Model file for the job. Use its own axes, mm. A direction names the side the tool comes from. Round coordinates to 2 decimals unless told otherwise and drop trailing zeros. Order: outer loops, then holes, each group sorted by start corner. A loop starts at its lowest first (then second) coordinate and runs counter-clockwise, first axis right, second up. Notation, with made-up numbers: (43, -24.75) - (50, -24.75) arc R24 ccw to (50, -13.75) - close; hole circle Ø8 at (45.5, 10). An arc over 180 degrees is marked (long way). Write item = value, one per line.
```python
from build123d import *

# Parameters (mm, degrees)
ESQUISSE1_W               = 47
ESQUISSE1_H               = 23
BOSS_EXTRU_1_DEPTH        = 7.071067812
TROU_TARAUD_M1_4X0_32_D   = 1.1
ESQUISSE5_W               = 20
ESQUISSE5_H               = 15
ENL_V_MAT_EXTRU_1_DEPTH   = 7.071067812
ESQUISSE6_W               = 20
ESQUISSE6_H               = 10.927419914
BOSS_EXTRU_2_DEPTH        = 7.071067812
ESQUISSE9_W               = 7.071067812
ESQUISSE9_H               = 7.071067812
BOSS_EXTRU_5_DEPTH        = 27
ESQUISSE10_R              = 1.5
ENL_V_MAT_EXTRU_2_DEPTH   = 3
TROU_TARAUD_M5X0_81_D     = 4.2
TROU_TARAUD_M5X0_81_DEPTH = 15
TROU_TARAUD_M5X0_81_TIP   = 1.2618073


with BuildPart() as part:
    # Esquisse1 → Boss.-Extru.1 (new body)
    with BuildSketch(Plane.XY):
        Rectangle(ESQUISSE1_W, ESQUISSE1_H)
    extrude(amount=BOSS_EXTRU_1_DEPTH)

    # Trou taraudé M1.4x0.32 (through all)
    with Locations(Plane(origin=(-21, 8.5, 7.071067812), x_dir=(1, 0, 0), z_dir=(0, 0, 1))):
        with Locations((0, 0), (0, -17), (42, -17), (42, 0)):
            Hole(TROU_TARAUD_M1_4X0_32_D / 2)

    # Esquisse5 → Enlèv. mat.-Extru.1 (cut)
    with BuildSketch(Plane.XY.offset(7.071067812)):
        with Locations((0, -6.927419914)):
            Rectangle(ESQUISSE5_W, ESQUISSE5_H)
    extrude(amount=-ENL_V_MAT_EXTRU_1_DEPTH, mode=Mode.SUBTRACT)

    # Esquisse6 → Boss.-Extru.2 (add)
    with BuildSketch(Plane(origin=(0, 0, 0), x_dir=(-1, 0, 0), z_dir=(0, 0, -1))):
        with Locations((0, 6.036290043)):
            Rectangle(ESQUISSE6_W, ESQUISSE6_H)
    extrude(amount=-BOSS_EXTRU_2_DEPTH)

    # Esquisse9 → Boss.-Extru.5 (add)
    with BuildSketch(Plane(origin=(0, 11.5, 0), x_dir=(1, 0, 0), z_dir=(0, 1, 0))):
        with Locations((0, -3.535533906)):
            Rectangle(ESQUISSE9_W, ESQUISSE9_H)
    extrude(amount=BOSS_EXTRU_5_DEPTH)

    # Esquisse10 → Enlèv. mat.-Extru.2 (cut)
    with BuildSketch(Plane(origin=(0, 38.5, 0), x_dir=(1, 0, 0), z_dir=(0, 1, 0))):
        with Locations(Location((0, -3.535533906, 0), (0, 0, 270))):
            Circle(ESQUISSE10_R)
    extrude(amount=-ENL_V_MAT_EXTRU_2_DEPTH, mode=Mode.SUBTRACT)

    # Trou taraudé M5x0.81
    with Locations(Plane(origin=(0, 38.5, 3.535533906), x_dir=(0, 0, 1), z_dir=(0, 1, 0))):
        with Locations((0, 0)):
            Hole(TROU_TARAUD_M5X0_81_D / 2, depth=TROU_TARAUD_M5X0_81_DEPTH)
            with Locations((0, 0, -(TROU_TARAUD_M5X0_81_DEPTH + TROU_TARAUD_M5X0_81_TIP / 2))):  # 118° drill point
                Cone(0, TROU_TARAUD_M5X0_81_D / 2, TROU_TARAUD_M5X0_81_TIP, mode=Mode.SUBTRACT)


solid = part.part
```
1) Cut at A-A (x = 12). Write the cut outline in (y, z).
Conclusion:
outline = (-11.5, 0) - (11.5, 0) - (11.5, 7.07) - (-11.5, 7.07) - close
2) 3-axis set-ups, long thin cutter, end or side, ignore diameter. For faces 4 (the face through (3.536, 25, 4)), 5 (the face through (-10, -6, 4)), 6 (the face through (-3.536, 25, 4)): which of +Z, -Z, +X, -X, +Y, -Y reach the whole face in a straight line?
Conclusion:
face_4 = +Z, -Z, +X, +Y
face_5 = +Z, -Z, -Y
face_6 = +Z, -Z, -X, +Y
3) Mould opens along Y. For faces 1 (the face through (-21.25, 8.01, 3.49)), 2 (the face through (-13, 11.5, 3)), 3 (the face through (23.5, 0, 3)) say: +Y half, -Y half, draft (parallel to the pull), parting line (faces both ways), or undercut.
Conclusion:
face_1 = undercut
face_2 = +Y half
face_3 = draft
4) Flat gauge pins, fed straight in: pin 1 Ø1.3 at (x, y) = (-21, -8.5) entering from -Z; pin 2 Ø3.5 at (x, z) = (-12, 4) entering from +Y; pin 3 Ø4 at (y, z) = (21.5, 5) entering from -X; pin 4 Ø3.5 at (y, z) = (24.5, 2) entering from +X. Where does each tip first touch, or does it go through?
Conclusion:
pin_1 = 0
pin_2 = 11.5
pin_3 = -3.54
pin_4 = 3.54
5) Wall check: line 1 along Y through (x, z) = (21, 5.5); line 2 along Z through (x, y) = (0, 35); line 3 along X through (y, z) = (-7, 5.25). Give the ranges that are in metal, low to high.
Conclusion:
line_1 = -11.5 to -9.05, -7.95 to 7.95, 9.05 to 11.5
line_2 = 0 to 1.44, 5.64 to 7.07
line_3 = -23.5 to -10, 10 to 23.5
6) Cut at B-B (z = 5). Give the number of separate pieces and of enclosed holes in the cut face, and give its area (3 significant figures).
Conclusion:
separate_pieces = 1
enclosed_holes = 4
area = 981 mm^2
